Design review of the part built by this model. Coordinates are the model's own, in mm. Coordinates: 2 decimals unless noted, no trailing zeros. Write each loop counter-clockwise with the first axis right and the second up, starting at its lowest first coordinate (ties: lowest second). Pieces come first, ordered by that corner, then holes.
Q1. Take a section at B-B, the plane x = 18. Write out the cut boundary in (y, z).
Q2. Take a section at A-A, the plane y = 28. Write out the cut boundary in (x, z), plus the area to 3 significant figures.
Q3. For L1, parallel to Z at x = 19, y = 19.5; L2, parallel to X at y = 20.5, z = 2.85; L3, parallel to Y at x = -16.5, z = 2.75, list the stretches that pass through material, from the lowest coordinate up.
Q4. Take a section at C-C, the plane y = -33.55. Write out the cut boundary in (x, z).
Q5. For pin 1 Ø3 at (x, z) = (-20, 1) entering from -Y; pin 2 Ø4 at (x, y) = (19.5, 15.5) entering from +Z; pin 3 Ø1.5 at (y, z) = (-40.5, 2.5) entering from +X; pin 4 Ø1.5 at (x, y) = (-15.5, -19.5) entering from -Z, all flat-tipped, find the tip position at first contact; note any pin that passes through.
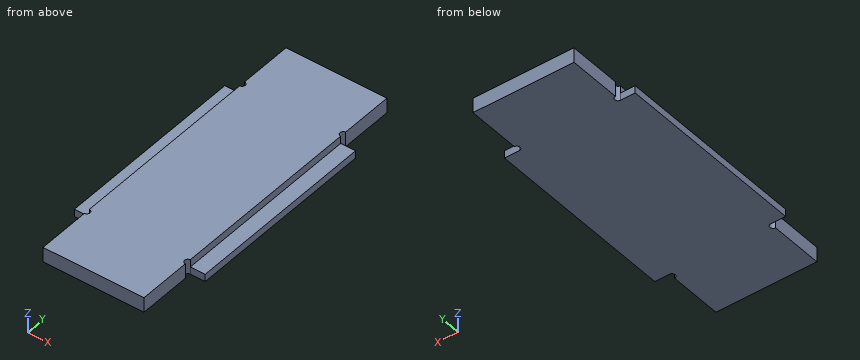
Autodesk Inventor part; units mm, degrees
ref_plane "YZ Plane" through (0, 0, 0) normal (1, 0, 0) x (0, 1, 0)
ref_plane "XZ Plane" through (0, 0, 0) normal (0, 1, 0) x (-1, 0, 0)
ref_plane "XY Plane" through (0, 0, 0) normal (0, 0, 1) x (1, 0, 0)
sketch "スケッチ1" plane through (0, 0, 0) normal (0, 0, 1) x (1, 0, 0)
  line L0 (-17, -52.5) -> (17, -52.5) construction
  line L1 (17, -52.5) -> (17, 52.5) construction
  line L2 (17, 52.5) -> (-17, 52.5) construction
  line L3 (-17, 52.5) -> (-17, -52.5) construction
  line L4 (-17, -52.5) -> (17, 52.5) construction
  line L5 (17, -52.5) -> (-17, 52.5) construction
  line L6 (-17, 34.6) -> (-17, 52.5)
  line L7 (-17, 52.5) -> (17, 52.5)
  line L8 (17, 52.5) -> (17, 34.6)
  line L9 (-17, -34.6) -> (-17, -52.5)
  line L10 (-17, -52.5) -> (17, -52.5)
  line L11 (17, -52.5) -> (17, -34.6)
  line L12 (-17, 32.5) -> (-22, 32.5)
  line L13 (-22, 32.5) -> (-22, -32.5)
  line L14 (-22, -32.5) -> (-17, -32.5)
  line L15 (17, 32.5) -> (22, 32.5)
  line L16 (22, 32.5) -> (22, -32.5)
  line L17 (22, -32.5) -> (17, -32.5)
  arc A0 (-17, 32.5) -> (-17, 34.6) centre (-17, 33.55) ccw
  arc A1 (-17, -34.6) -> (-17, -32.5) centre (-17, -33.55) ccw
  arc A2 (17, 34.6) -> (17, 32.5) centre (17, 33.55) ccw
  arc A3 (17, -32.5) -> (17, -34.6) centre (17, -33.55) ccw
  line L18 (0, 0) -> (17, 0) construction
  line L19 (0, 0) -> (0, 52.5) construction
  line L20 (-12, 42.5) -> (12, 42.5) construction
  line L21 (12, 42.5) -> (12, -42.5) construction
  line L22 (12, -42.5) -> (-12, -42.5) construction
  line L23 (-12, -42.5) -> (-12, 42.5) construction
  circle A4 centre (-12, 42.5) radius 1.2
  circle A5 centre (12, 42.5) radius 1.2
  circle A6 centre (12, -42.5) radius 1.2
  circle A7 centre (-12, -42.5) radius 1.2
  point P0 (0, 42.5)
  point P1 (0, 0)
  dimension "d87" = 1.05
  dimension "d88" = 105
  dimension "d89" = 5
  dimension "d90" = 20
  dimension "d91" = 34
  dimension "d92" = 2.4
  dimension "d93" = 5
  dimension "d94" = 10
  dimension "d95" = 10
extrude "押し出し1" add sketch "スケッチ1" along normal blind 5
sketch "スケッチ2" plane through (0, 0, 5) normal (0, 0, 1) x (1, 0, 0)
  line L0 (-17, 52.5) -> (-17, 34.6)
  line L1 (17, 34.6) -> (17, 52.5)
  line L2 (-40.5884, 60.19) -> (-17, 60.19)
  line L3 (-17, 60.19) -> (-17, -101.7483)
  line L4 (-17, -101.7483) -> (-40.5884, -101.7483)
  line L5 (-40.5884, -101.7483) -> (-40.5884, 60.19)
  line L6 (53.5752, 90.4043) -> (17, 90.4043)
  line L7 (17, 90.4043) -> (17, -93.5321)
  line L8 (17, -93.5321) -> (53.5752, -93.5321)
  line L9 (53.5752, -93.5321) -> (53.5752, 90.4043)
  point P0 (0, 0)
extrude "押し出し2" cut sketch "スケッチ2" against normal blind 2.5
sketch "スケッチ4" plane through (0, 0, 5) normal (0, 0, 1) x (1, 0, 0)
  circle A0 centre (-12, -42.5) radius 1.2
  circle A1 centre (-12, -42.5) radius 1.2
  circle A2 centre (12, -42.5) radius 1.2
  circle A3 centre (12, -42.5) radius 1.2
  circle A4 centre (-12, 42.5) radius 1.2
  circle A5 centre (-12, 42.5) radius 1.2
  circle A6 centre (12, 42.5) radius 1.2
  circle A7 centre (12, 42.5) radius 1.2
  point P0 (0, 0)
extrude "押し出し4" add sketch "スケッチ4" against normal up to surface (5 mm away)
equation "\"d88\" = d83"
equation "\"d90\" = d84"
properties part number "コックピット_2_サブフレーム_5" material "アセタール樹脂、黒"
Responses:
1. outline: (-32.5, 0) - (32.5, 0) - (32.5, 2.5) - (-32.5, 2.5) - close
2. outline: (-22, 0) - (22, 0) - (22, 2.5) - (17, 2.5) - (17, 5) - (-17, 5) - (-17, 2.5) - (-22, 2.5) - close
2. area: 195 mm2
3. L1: z = 0 to 2.5
3. L2: x = -17 to 17
3. L3: y = -52.5 to -34.47, -32.63 to 32.63, 34.47 to 52.5
4. outline: (-15.95, 0) - (15.95, 0) - (15.95, 5) - (-15.95, 5) - close
5. pin 1: stops at y = -32.5
5. pin 2: stops at z = 2.5
5. pin 3: stops at x = 17
5. pin 4: stops at z = 0
